The listing builds one solid part. Answer for the finished solid, in the listing's coordinates (mm). A direction names the side the tool comes from. Round coordinates to 2 decimals unless told otherwise and drop trailing zeros. Write each loop counter-clockwise with the first axis right and the second up, starting at its lowest first coordinate (ties: lowest second). Pieces come first, ordered by that corner, then holes. Notation, with made-up numbers: (54, 62) -> (64, 62) arc R9 ccw to (64, 67) -> close; hole circle Ø4 at (16.5, 46). An arc over 180 degrees is marked (long way). Write each question's results on one line, items separated by ' | '. Start each with the question number.
```python
from build123d import *

# Parameters (mm, degrees)
F1_DEPTH = 12.7


with BuildPart() as f1:
    # F0 (on Top) → F1 (new body)
    with BuildSketch(Plane.XY):
        with BuildLine():
            Line((0, 28.575), (0, 38.1))
            ThreePointArc((0, 38.1), (-23.865153, 17.334725), (-24.746676, -14.2875))
            Line((-24.746676, -14.2875), (-32.995568, -19.05))
            ThreePointArc((-32.995568, -19.05), (-3.079736, -29.335191), (24.746676, -14.2875))
            Line((24.746676, -14.2875), (32.995568, -19.05))
            ThreePointArc((32.995568, -19.05), (26.944888, 12.000466), (0, 28.575))
        make_face()
        Polygon((0, 10.998523), (9.525, 5.499261), (9.525, -5.499261), (0, -10.998523), (-9.525, -5.499261), (-9.525, 5.499261), align=None, mode=Mode.SUBTRACT)
    extrude(amount=F1_DEPTH)


solid = f1.part
```
Q1. For faces 4 (the flat face through (28.813, -16.635, 6.261)), 5 (the flat face through (-28.813, -16.635, 6.261)), 6 (the flat face through (9.525, 0, 6)), determine the directions among +Z, -Z, +X, -X, +Y, -Y from which every point of the face is accessible in a straight line to the end or side of a thin tool.
Q2. Determine the mould class of faces 1 (the flat face through (0, 33, 6)), 2 (the flat face through (0, 12, 12.7)), 3 (the flat face through (-4.83, 8.21, 6.26)) for opening direction X: pulls with the +X half, pulls with the -X half, needs draft (parallel to the pull), parting line crosses it, or undercut.
Q3. Each of these flat-tipped pins is pushed along its axis until it touches: pin 1 (1.5 mm diameter, centred on y = -4.5, z = 2.5, fed in from +X); pin 2 (2 mm diameter, centred on x = -22, z = 9, fed in from -Y); pin 3 (6 mm diameter, centred on x = -16, z = 5, fed in from -Y). Where does it stop, or does it pass through?
Q4. Find the intervals of material crossed by line 1 (Y direction, x = 8, z = 8); line 2 (X direction, y = -16.5, z = 5.25); line 3 (Y direction, x = 7.5, z = 9.5), in increasing order.
Q5. The part is cut by section D-D, the plane y = 26. Write down the section's boundary in (x, z).
Q6. The part is cut by section B-B, the plane x = -26. Write down the section's boundary in (y, z), then the cut area to 3 significant figures.
Q7. The part is cut by section A-A, the plane y = -6.5. Write down the section's boundary in (x, z), then the cut area to 3 significant figures.
Answers follow:
1) face 4: +Z, -Z, -Y | face 5: +Z, -Z, -X | face 6: +Z, -Z
2) face 1: pulls with the +X half | face 2: needs draft | face 3: undercut
3) pin 1: x = 33.61 | pin 2: y = -26.63 | pin 3: y = -28.9
4) line 1: -26.77 to -6.38, 6.38 to 26.59 | line 2: -28.58 to 22.89, 28.58 to 33.48 | line 3: -26.96 to -6.67, 6.67 to 26.77
5) outline: (-18.28, 0) -> (9.53, 0) -> (9.53, 12.7) -> (-18.28, 12.7) -> close
6) outline: (-24.19, 0) -> (-15.01, 0) -> (-15.01, 12.7) -> (-24.19, 12.7) -> close; (-10.72, 0) -> (11.75, 0) -> (11.75, 12.7) -> (-10.72, 12.7) -> close | area: 402 mm^2
7) outline: (-27.01, 0) -> (-7.79, 0) -> (-7.79, 12.7) -> (-27.01, 12.7) -> close; (7.79, 0) -> (33.76, 0) -> (33.76, 12.7) -> (7.79, 12.7) -> close | area: 574 mm^2
